Read the model definition and answer for the solid it produces. Units are mm, in the model's axes. Face numbers are marked on the shaded views. A direction names the side the tool comes from. Round coordinates to 2 decimals unless told otherwise and drop trailing zeros. Loops run counter-clockwise (first coordinate to the right, second up) from the corner with the lowest first, then second, coordinate; pieces in that order, holes last. Notation, with made-up numbers: M 27,-10 L 59,-10 A20 cw 59,10 Z; hole C 53.5,-18 d2. An arc over 180 degrees is marked long. Write each question's results on one line, items separated by ' | '.
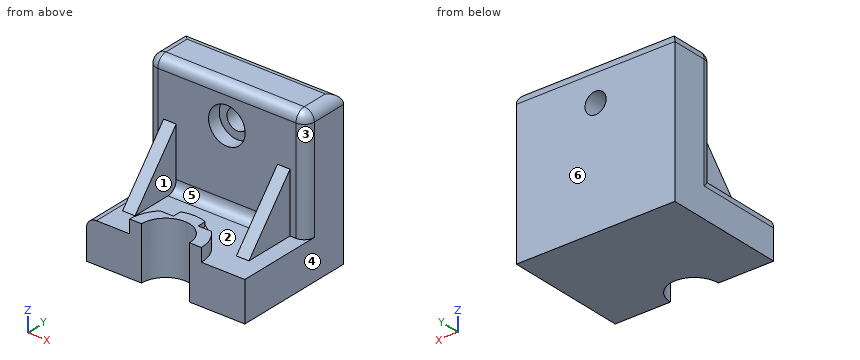
```python
from build123d import *

# Parameters (mm, degrees)
F1_DEPTH  = 79.248
F2_W      = 6.267937
F2_H      = 29.795837
F3_DEPTH  = 25.4
F4_DEPTH  = 25.4
F6_DEPTH  = 25.4
F7_DEPTH  = 6.604
F9_DEPTH  = 25.4
F11_DEPTH = 25.4
F2_R      = 5.269734
F12_DEPTH = 25.4
F2_R_2    = 9.158021
F13_DEPTH = 6.604
F14_R     = 5.08


with BuildPart() as f1:
    # F0 (on Right) → F1 (new body)
    with BuildSketch(Plane.YZ):
        Polygon((33.579409, 56.474458), (10.37909, 56.474458), (10.37909, 0), (-27.474059, 0), (-27.474059, -19.842375), (33.579409, -19.842375), align=None)
    extrude(amount=F1_DEPTH)

    # F2 (on face) → F3 (join)
    with BuildSketch(Plane.XZ.offset(-10.37909)):
        with Locations((11.170426, 14.897918)):
            Rectangle(F2_W, F2_H)
    extrude(amount=F3_DEPTH)

    # F2 (on face) → F4 (join)
    with BuildSketch(Plane.XZ.offset(-10.37909)):
        with Locations((68.077574, 14.897918)):
            Rectangle(F2_W, F2_H)
    extrude(amount=F4_DEPTH)

    # F5 (on face) → F6 (cut)
    with BuildSketch(Plane.XY):
        with BuildLine():
            ThreePointArc((51.611442, -27.474059), (39.624, -15.486617), (27.636558, -27.474059))
            Line((27.636558, -27.474059), (51.611442, -27.474059))
        make_face()
    extrude(amount=-F6_DEPTH, mode=Mode.SUBTRACT)

    # F5 (on face) → F7 (join)
    with BuildSketch(Plane.XY):
        with BuildLine():
            Line((21.696024, -27.474059), (27.636558, -27.474059))
            ThreePointArc((27.636558, -27.474059), (39.624, -15.486617), (51.611442, -27.474059))
            Line((51.611442, -27.474059), (57.551976, -27.474059))
            ThreePointArc((57.551976, -27.474059), (39.624, -9.546082), (21.696024, -27.474059))
        make_face()
    extrude(amount=F7_DEPTH)

    # F8 (on face) → F9 (cut)
    with BuildSketch(Plane.YZ.offset(71.211543)):
        Polygon((-15.02091, 0), (10.37909, 29.795837), (-15.02091, 29.795837), align=None)
    extrude(amount=-F9_DEPTH, mode=Mode.SUBTRACT)

    # F10 (on face) → F11 (cut)
    with BuildSketch(Plane(origin=(8.036457, 0, 0), x_dir=(0, -1, 0), z_dir=(-1, 0, 0))):
        Polygon((15.02091, 29.795837), (-10.37909, 29.795837), (15.02091, 0), align=None)
    extrude(amount=-F11_DEPTH, mode=Mode.SUBTRACT)

    # F2 (on face) → F12 (cut)
    with BuildSketch(Plane.XZ.offset(-10.37909)):
        with Locations((39.624, 38.005784)):
            Circle(F2_R)
    extrude(amount=-F12_DEPTH, mode=Mode.SUBTRACT)

    # F2 (on face) → F13 (cut)
    with BuildSketch(Plane.XZ.offset(-10.37909)):
        with Locations((39.624, 38.005784)):
            Circle(F2_R_2)
        with Locations((39.624, 38.005784)):
            Circle(F2_R, mode=Mode.SUBTRACT)
    extrude(amount=-F13_DEPTH, mode=Mode.SUBTRACT)

    # F14
    f14_edges = [f1.edges().sort_by_distance(p)[0] for p in [
        (0, 21.97925, 56.474458),
        (79.248, 21.97925, 56.474458),
        (0, -8.547484, 0),
        (0, 10.37909, 28.237229),
        (39.624, 10.37909, 56.474458),
        (39.624, 33.579409, 56.474458),
        (79.248, 10.37909, 28.237229),
        (39.624, 10.37909, 0),
    ]]
    fillet(f14_edges, radius=F14_R)


solid = f1.part
```
1. Which of the six approach directions +Z, -Z, +X, -X, +Y, -Y give full straight-line access (tool end or side, diameter ignored) to the marked faces 1, 2 and 3?
Completed:
face 1: +Z, -Y | face 2: +Z | face 3: +Z, +X, -Y
2. Given P1, Ø12.5, axis at y = -7.5, z = 13.5, coming from the +X side; P2, Ø19.5, axis at x = 31, y = -20.5, coming from the +Z side; P3, Ø20.5, axis at y = 0, z = 18, coming from the -X side; P4, Ø12, axis at x = 39.62, z = 38.01, coming from the +Y side, each flat-ended and moving along its own axis, determine where each tip first touches the part or whether it passes through.
Completed:
P1: stops at x = 71.21 | P2: stops at z = 6.6 | P3: stops at x = 8.04 | P4: stops at y = 33.58
3. Determine the mould class of the marked faces 4, 5 and 6 for opening direction Y: released by +Y, released by -Y, zero draft, split by the parting line, or undercut.
Completed:
face 4: zero draft | face 5: undercut | face 6: released by +Y
4. Find section D-D, the plane x = 62. Give the vertices of the cut face in (y, z), then the cut area to 3 significant figures.
Completed:
outline: M -27.47,-19.84 L 33.58,-19.84 L 33.58,51.39 A5.08 ccw 28.5,56.47 L 15.46,56.47 A5.08 ccw 10.38,51.39 L 10.38,5.08 A5.08 cw 5.3,0 L -27.47,0 Z | area: 2,520 mm2
5. Find section C-C, the plane z = -11. Give the vertices of the cut face in (x, y).
Completed:
outline: M 0,-27.47 L 27.64,-27.47 A11.99 cw 51.61,-27.47 L 79.25,-27.47 L 79.25,33.58 L 0,33.58 Z
6. Find section A-A, the plane x = 42. Give the vertices of the cut face in (y, z).
Completed:
outline: M -15.72,-19.84 L 33.58,-19.84 L 33.58,33.3 L 16.98,33.3 L 16.98,29.16 L 10.38,29.16 L 10.38,5.08 A5.08 cw 5.3,0 L -9.7,0 L -9.7,6.6 L -15.72,6.6 Z; M 10.38,46.85 L 16.98,46.85 L 16.98,42.71 L 33.58,42.71 L 33.58,51.39 A5.08 ccw 28.5,56.47 L 15.46,56.47 A5.08 ccw 10.38,51.39 Z
7. Find the intervals of material crossed by L1, parallel to Z at x = 61, y = -4.5; L2, parallel to Y at x = 59, z = 8; L3, parallel to X at y = 1, z = 1.5, in increasing order.
Completed:
L1: z = -19.84 to 0 | L2: y = 10.38 to 33.58 | L3: x = 8.04 to 14.3, 64.94 to 71.21
8. Find section B-B, the plane y = -16.5. Give the vertices of the cut face in (x, z).
Completed:
outline: M 0,-19.84 L 34.8,-19.84 L 34.8,6.6 L 25.45,6.6 L 25.45,0 L 5.08,0 A5.08 ccw 0,-5.08 Z; M 44.45,-19.84 L 79.25,-19.84 L 79.25,0 L 53.8,0 L 53.8,6.6 L 44.45,6.6 Z
